Design review of the part built by this model. Coordinates are the model's own, in mm. Face numbers are marked on the shaded views. A direction names the side the tool comes from. Give positions to 0.01 mm unless a question says otherwise; leave off trailing zeros. Write each loop counter-clockwise with the first axis right and the second up, starting at its lowest first coordinate (ties: lowest second). Pieces come first, ordered by that corner, then holes. Notation, with made-up numbers: (63, 80.5) - (101, 80.5) arc R6 ccw to (101, 88.5) - close; hole circle Ø7 at (-20, 80.25). An arc over 180 degrees is marked (long way). Use a Markdown table: item, result. Add a question column.
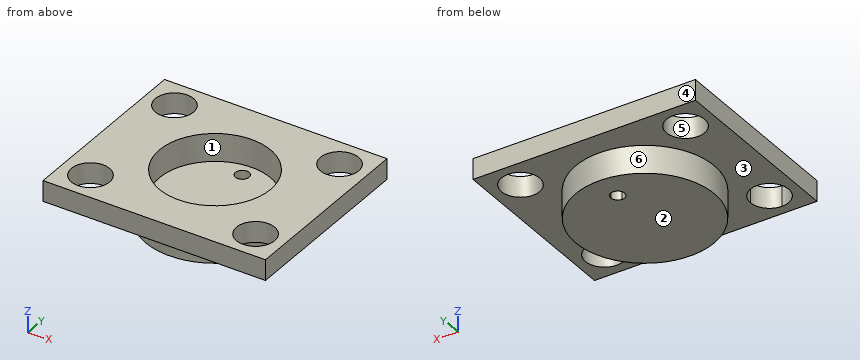
```python
from build123d import *

# Parameters (mm, degrees)
F0_R     = 7.9121
F1_DEPTH = 3.175
F2_W     = 25.4
F2_H     = 21.209
F3_DEPTH = 2.3622
F4_R     = 6.35
F5_DEPTH = 3.175
F7_DEPTH = 2.3632
F8_R     = 2.18313
F9_DEPTH = 5.5382


with BuildPart() as f1:
    # F0 (on Top) → F1 (new body)
    with BuildSketch(Plane.XY):
        Circle(F0_R)
    extrude(amount=F1_DEPTH)

    # F2 (on face) → F3 (join)
    with BuildSketch(Plane.XY.offset(3.175)):
        Rectangle(F2_W, F2_H)
    extrude(amount=F3_DEPTH)

    # F4 (on face) → F5 (cut)
    with BuildSketch(Plane.XY.offset(5.5372)):
        Circle(F4_R)
    extrude(amount=-F5_DEPTH, mode=Mode.SUBTRACT)

    # F6 (on face) → F7 (cut, through all)
    with BuildSketch(Plane.XY.offset(2.3622)):
        with BuildLine():
            ThreePointArc((0, 3.9751), (0.556776, 4.205724), (0.7874, 4.7625))
            ThreePointArc((0.7874, 4.7625), (-0.556776, 5.319276), (0, 3.9751))
        make_face()
    extrude(amount=-F7_DEPTH, mode=Mode.SUBTRACT)

    # F8 (on face) → F9 (cut, through all)
    with BuildSketch(Plane.XY.offset(5.5372)):
        with Locations((9.42467, 7.32917)):
            Circle(F8_R)
        with BuildLine():
            ThreePointArc((-11.6078, 7.32917), (-9.42467, 5.14604), (-7.24154, 7.32917))
            ThreePointArc((-7.24154, 7.32917), (-9.42467, 9.5123), (-11.6078, 7.32917))
        make_face()
        with BuildLine():
            ThreePointArc((-9.42467, -9.5123), (-7.880964, -8.872876), (-7.24154, -7.32917))
            ThreePointArc((-7.24154, -7.32917), (-10.968376, -5.785464), (-9.42467, -9.5123))
        make_face()
        with Locations((9.42467, -7.32917)):
            Circle(F8_R)
    extrude(amount=-F9_DEPTH, mode=Mode.SUBTRACT)


solid = f1.part
```
(1) Add section B-B (y = -5.5). State the section outline as (x, z) points (3 decimals).
(2) Tool access review of the marked faces 1, 2 and 3: name each direction out of +Z, -Z, +X, -X, +Y, -Y from which nothing blocks a thin tool from reaching the whole face with its end or side.
(3) Insertion check: pin 1 (5 mm diameter, centred on x = -9.42, y = -7.33, fed in from -Z) (3 decimals); pin 2 (1.8 mm diameter, centred on x = 0, y = 4.76, fed in from +Z). Each pin has a flat end and moves straight along its axis. Give the tip position at first contact, or say it passes through.
(4) Add section C-C (x = -4.5). State the section outline as (y, z) points (1 decimal), and give its area (3 significant figures).
(5) For line 1 along X through (y, z) = (7.5, 4); line 2 along Y through (x, z) = (9.5, 4.05); line 3 along Y through (x, z) = (0, 3.65), list the stretches that pass through material, from the lowest coordinate up.
(6) Add section A-A (z = 2.75). State the section outline as (x, y) points.
(7) Mouldability with a two-part tool opening along X and no side actions: class the marked faces 4, 5 and 6 as +X half, -X half, draft (parallel to the pull), parting line (faces both ways), or undercut.
(8) Add section D-D (y = 0). State the section outline as (x, z) points (3 decimals).
Answers follow:
| question | item | result |
|---|---|---|
| 1 | outline | (-12.7, 3.175) - (-10.616, 3.175) - (-10.616, 5.537) - (-12.7, 5.537) - close; (-8.233, 3.175) - (-5.688, 3.175) - (-5.688, 0) - (5.688, 0) - (5.688, 3.175) - (8.233, 3.175) - (8.233, 5.537) - (3.174, 5.537) - (3.174, 2.362) - (-3.174, 2.362) - (-3.174, 5.537) - (-8.233, 5.537) - close; (10.616, 3.175) - (12.7, 3.175) - (12.7, 5.537) - (10.616, 5.537) - close |
| 2 | face 1 | +Z |
| 2 | face 2 | -Z, +X, -X, +Y, -Y |
| 2 | face 3 | -Z |
| 3 | pin 1 | z = 3.175 |
| 3 | pin 2 | z = 2.36 |
| 4 | outline | (-10.6, 3.2) - (-6.5, 3.2) - (-6.5, 0) - (6.5, 0) - (6.5, 3.2) - (10.6, 3.2) - (10.6, 5.5) - (4.5, 5.5) - (4.5, 2.4) - (-4.5, 2.4) - (-4.5, 5.5) - (-10.6, 5.5) - close |
| 4 | area | 63.0 mm^2 |
| 5 | line 1 | -12.7 to -11.6, -7.25 to 7.25, 11.6 to 12.7 |
| 5 | line 2 | -10.6 to -9.51, -5.15 to 5.15, 9.51 to 10.6 |
| 5 | line 3 | -10.6 to -6.35, 6.35 to 10.6 |
| 6 | outline | circle Ø15.82 at (0, 0); hole circle Ø12.7 at (0, 0) |
| 7 | face 4 | draft |
| 7 | face 5 | undercut |
| 7 | face 6 | parting line |
| 8 | outline | (-12.7, 3.175) - (-7.912, 3.175) - (-7.912, 0) - (7.912, 0) - (7.912, 3.175) - (12.7, 3.175) - (12.7, 5.537) - (6.35, 5.537) - (6.35, 2.362) - (-6.35, 2.362) - (-6.35, 5.537) - (-12.7, 5.537) - close |
